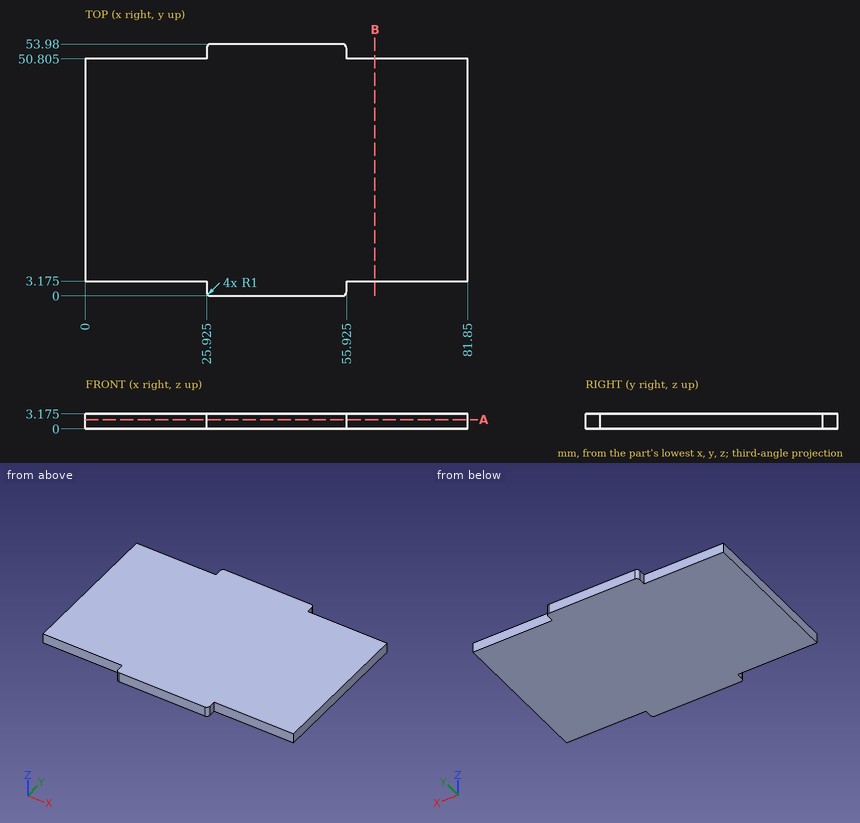
Here's the drawing with two shaded views (mm, measured from the low corner). I have some questions. Give positions to 0.01 mm unless a question says otherwise; leave off trailing zeros. Order: outer loops, then holes, each group sorted by start corner. A loop starts at its lowest first (then second) coordinate and runs counter-clockwise, first axis right, second up. Notation, with made-up numbers: M -15.75,-32.5 L 35.25,-32.5 A16 ccw 35.25,-21.5 Z; hole C 33.25,-23.5 d8. An arc over 180 degrees is marked long. One line per item, written item: value.
1) I want a section at B-B, the plane x = 62. List the corners of the cut face in (y, z) for me (3 decimals).
Answer sheet:
outline: M 3.175,0 L 50.805,0 L 50.805,3.175 L 3.175,3.175 Z
2) Please list where this line runs through material, in increasing order: line 1 along Y through (x, z) = (11, 1.15) (3 decimals).
Answer sheet:
line 1: y = 3.175 to 50.805
3) I want a section at A-A, the plane z = 1.95. List the corners of the cut face in (x, y) for me (3 decimals), plus the area to 3 significant figures.
Answer sheet:
outline: M 0,3.175 L 25.925,3.175 L 25.925,1 A1 ccw 26.925,0 L 54.925,0 A1 ccw 55.925,1 L 55.925,3.175 L 81.85,3.175 L 81.85,50.805 L 55.925,50.805 L 55.925,52.98 A1 ccw 54.925,53.98 L 26.925,53.98 A1 ccw 25.925,52.98 L 25.925,50.805 L 0,50.805 Z
area: 4,090 mm^2
4) For P1, Ø1.7, axis at y = 2, z = 1.5, coming from the -X side (3 decimals); P2, Ø1, axis at x = 63, z = 1, coming from the +Y side (3 decimals), each with a flat end and sliding along its axis, tell me the tip position at first contact or that it passes through.
Answer sheet:
P1: stops at x = 25.925
P2: stops at y = 50.805
